Part model, mm, in its own coordinate system. Face numbers are marked on the shaded views. A direction names the side the tool comes from. Coordinates: 2 decimals unless noted, no trailing zeros. Loops run counter-clockwise (first coordinate to the right, second up) from the corner with the lowest first, then second, coordinate; pieces in that order, holes last. Notation, with made-up numbers: M 31.25,-37 L 74.25,-37 A15 ccw 74.25,-22 Z; hole C 0.25,61.25 d8. An arc over 180 degrees is marked long. Answer as a JSON object with one key per item and string values. Group by question number.
1. Mould opens along Z. For the marked faces 1, 2, 3 and 4 say: released by +Z, released by -Z, zero draft, split by the parting line, or undercut.
2. 3-axis set-ups, long thin cutter, end or side, ignore diameter. For the marked faces 5, 6 and 7: which of +Z, -Z, +X, -X, +Y, -Y reach the whole face in a straight line?
3. Saw through at B-B on x = 0. Write the cut outline in (y, z), then the cut area to 3 significant figures.
4. Saw through at D-D on z = 2. Write the cut outline in (x, y).
5. Saw through at A-A on y = 0. Write the cut outline in (x, z).
6. Drop a flat-ended pin along its axis: pin 1 Ø1.9 at (y, z) = (10, 1) entering from +X. Give the stop position or say it passes through.
7. Saw through at C-C on x = 3. Write the cut outline in (y, z).
8. Drill centre lines: L1, parallel to Z at x = -1.5, y = 0; L2, parallel to Z at x = -0.75, y = -5.5; L3, parallel to Y at x = -1.5, z = 0.25. Where is each one in solid material? Low to high.
from build123d import *

# Parameters (mm, degrees)
PAD013_DEPTH            = 1.1
PAD014_DEPTH            = 1.75
PAD014_DEPTH_BACK       = 1.75
PAD015_DEPTH            = 1.1
BODY008_PLACEMENT_ANGLE = 90


with BuildPart() as part:
    # Sketch022 → Pad013 (new body)
    with BuildSketch(Plane.XY):
        with BuildLine():
            ThreePointArc((-4.41588, -1.75), (-0.373115, -4.735323), (4.08731, -2.42))
            Line((4.08731, -2.42), (8.306624, -2.75))
            ThreePointArc((8.306624, -2.75), (10.107666, 0), (8.306624, 2.75))
            Line((4.08731, 2.42), (8.306624, 2.75))
            ThreePointArc((4.08731, 2.42), (-0.373115, 4.735323), (-4.41588, 1.75))
            Line((-4.41588, -1.75), (-4.41588, 1.75))
        make_face()
    extrude(amount=PAD013_DEPTH)

    # Sketch023 → Pad014 (join, two sides)
    with BuildSketch(Plane.XZ) as pad014_sk:
        with BuildLine():
            ThreePointArc((-9.41588, 0), (-11.41588, -2), (-9.41588, -4))
            Line((-9.41588, -4), (-4.41588, -4))
            Line((-4.41588, -4), (-4.41588, -5.1))
            Line((-9.41588, -5.1), (-4.41588, -5.1))
            ThreePointArc((-9.41588, 1.1), (-12.51588, -2), (-9.41588, -5.1))
            Line((-4.41588, 1.1), (-9.41588, 1.1))
            Line((-4.41588, 1.1), (-4.41588, 0))
            Line((-9.41588, 0), (-4.41588, 0))
        make_face()
    extrude(amount=PAD014_DEPTH)
    extrude(pad014_sk.sketch, amount=-PAD014_DEPTH_BACK)

    # Sketch025 (on Face9 of Pad014) → Pad015 (join)
    with BuildSketch(Plane.XY.offset(-4)):
        with BuildLine():
            ThreePointArc((-4.41588, -1.75), (4.75, 0), (-4.41588, 1.75))
            Line((-4.41588, 1.75), (-4.41588, -1.75))
        make_face()
    extrude(amount=-PAD015_DEPTH)


with BuildPart() as part_1:
    # Body008 placement: moved
    add(part.part.moved(Location((0, 0, 4))).rotate(Axis((0, 0, 4), (0, 0, -1)), BODY008_PLACEMENT_ANGLE))


solid = part_1.part
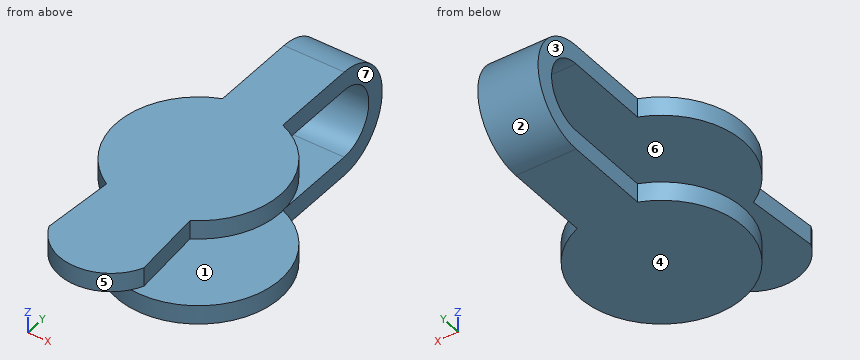
Outcome:
{
 "1": {"face 1": "undercut", "face 2": "split by the parting line", "face 3": "zero draft", "face 4": "released by -Z"},
 "2": {"face 5": "+Z, -Z, -Y", "face 6": "+X, -X, -Y", "face 7": "+Z, -Z, +X, +Y"},
 "3": {"outline": "M -10.11,4 L 9.42,4 A2 cw 9.42,0 L -4.75,0 L -4.75,-1.1 L 9.42,-1.1 A3.1 ccw 9.42,5.1 L -10.11,5.1 Z", "area": "45.9 mm²"},
 "4": {"outline": "M -1.75,11.42 L 1.75,11.42 L 1.75,12.52 L -1.75,12.52 Z"},
 "5": {"outline": "M -4.75,-1.1 L 4.75,-1.1 L 4.75,0 L -4.75,0 Z; M -4.75,4 L 4.75,4 L 4.75,5.1 L -4.75,5.1 Z"},
 "6": {"pin 1": "stops at x = 1.75"},
 "7": {"outline": "M -3.68,-1.1 L 3.68,-1.1 L 3.68,0 L -3.68,0 Z; M -3.68,4 L 3.68,4 L 3.68,5.1 L -3.68,5.1 Z"},
 "8": {"L1": "z = -1.1 to 0, 4 to 5.1", "L2": "z = 4 to 5.1", "L3": "y = 10.38 to 11.97"}
}
